Check sheet for the modelled part. Datum: model origin and axes. Units: mm. A direction names the side the tool comes from. Round coordinates to 2 decimals unless told otherwise and drop trailing zeros. Write each loop counter-clockwise with the first axis right and the second up, starting at its lowest first coordinate (ties: lowest second). Pieces come first, ordered by that corner, then holes. Notation, with made-up numbers: M 77,71.25 L 115,71.25 A19 ccw 115,96.25 Z; hole C 51.5,67 d3. An arc over 180 degrees is marked long. One line per item, written item: value.
from build123d import *

# Parameters (mm, degrees)
SKETCH2_W           = 90
SKETCH2_H           = 50
BOSS_EXTRUDE2_DEPTH = 5
SKETCH4_R           = 1
BOSS_EXTRUDE3_DEPTH = 4
SKETCH5_R           = 2
CUT_EXTRUDE1_DEPTH  = 18


with BuildPart() as part:
    # Sketch2 → Boss-Extrude2 (new body)
    with BuildSketch(Plane(origin=(0, 0, 0), x_dir=(1, 0, 0), z_dir=(0, 1, 0))):
        with Locations((-113.562992126, 38.956692913)):
            Rectangle(SKETCH2_W, SKETCH2_H)
    extrude(amount=BOSS_EXTRUDE2_DEPTH)

    # Sketch4 → Boss-Extrude3 (add)
    with BuildSketch(Plane(origin=(0, 5, 0), x_dir=(1, 0, 0), z_dir=(0, 1, 0))):
        with Locations(Location((-145.062992126, 22.456692913, 0), (0, 0, 270))):
            Circle(SKETCH4_R)
        with Locations(Location((-145.062992126, 55.456692913, 0), (0, 0, 270))):
            Circle(SKETCH4_R)
        with Locations(Location((-82.062992126, 55.456692913, 0), (0, 0, 270))):
            Circle(SKETCH4_R)
        with Locations(Location((-82.062992126, 22.456692913, 0), (0, 0, 270))):
            Circle(SKETCH4_R)
    extrude(amount=BOSS_EXTRUDE3_DEPTH)

    # Sketch5 → Cut-Extrude1 (cut)
    with BuildSketch(Plane.XZ):
        with Locations(Location((-113.562992126, -38.956692913, 0), (0, 0, 270))):
            Circle(SKETCH5_R)
    extrude(amount=-CUT_EXTRUDE1_DEPTH, mode=Mode.SUBTRACT)


solid = part.part
Q1. Scan lines: line 1 (Y direction, x = -119, z = -32); line 2 (Z direction, x = -112.5, y = 1.5); line 3 (X direction, y = 3, z = -38.5). Record each from-to range of solid material in increasing order. Write a range as [from, to].
Completed:
line 1: [0, 5]
line 2: [-63.96, -40.65], [-37.26, -13.96]
line 3: [-158.56, -115.51], [-111.62, -68.56]
Q2. Sectioned sample at B-B on x = -84. Enter the section's corners in (y, z), and give its area (3 significant figures).
Completed:
outline: M 0,-63.96 L 5,-63.96 L 5,-13.96 L 0,-13.96 Z
area: 250 mm^2
Q3. Depth check by flat-ended pin: P1, Ø25, axis at x = -109, z = -31.5, coming from the +Y side. Enter the tip coordinate at first touch or a pass-through.
Completed:
P1: y = 5
Q4. Sectioned sample at A-A on z = -30. Enter the section's corners in (x, y), and give its area (3 significant figures).
Completed:
outline: M -158.56,0 L -68.56,0 L -68.56,5 L -158.56,5 Z
area: 450 mm^2
Q5. Access from +Z, -Z, +X, -X, +Y, -Y to the whole of each face (thin tool, end or side, straight path). Record for faces 1 (the cylindrical face through (-81.07, 6.97, -22.59)), 2 (the flat face through (-145, 9, -55)).
Completed:
face 1: +Y
face 2: +Z, -Z, +X, -X, +Y
Q6. Draft check along Z on faces 3 (the flat face through (-82, 9, -22)), 4 (the cylindrical face through (-81.22, 6.97, -54.92)), 5 (the flat face through (-114, 2, -63.957)). Enter one of: pulls with the +Z half, pulls with the -Z half, needs draft (parallel to the pull), parting line crosses it, or undercut.
Completed:
face 3: needs draft
face 4: undercut
face 5: pulls with the -Z half
Q7. Sectioned sample at C-C on y = 7.25. Enter the section's corners in (x, z), and give its area (3 significant figures).
Completed:
outline: C -145.06,-55.46 d2; C -145.06,-22.46 d2; C -82.06,-55.46 d2; C -82.06,-22.46 d2
area: 12.6 mm^2
